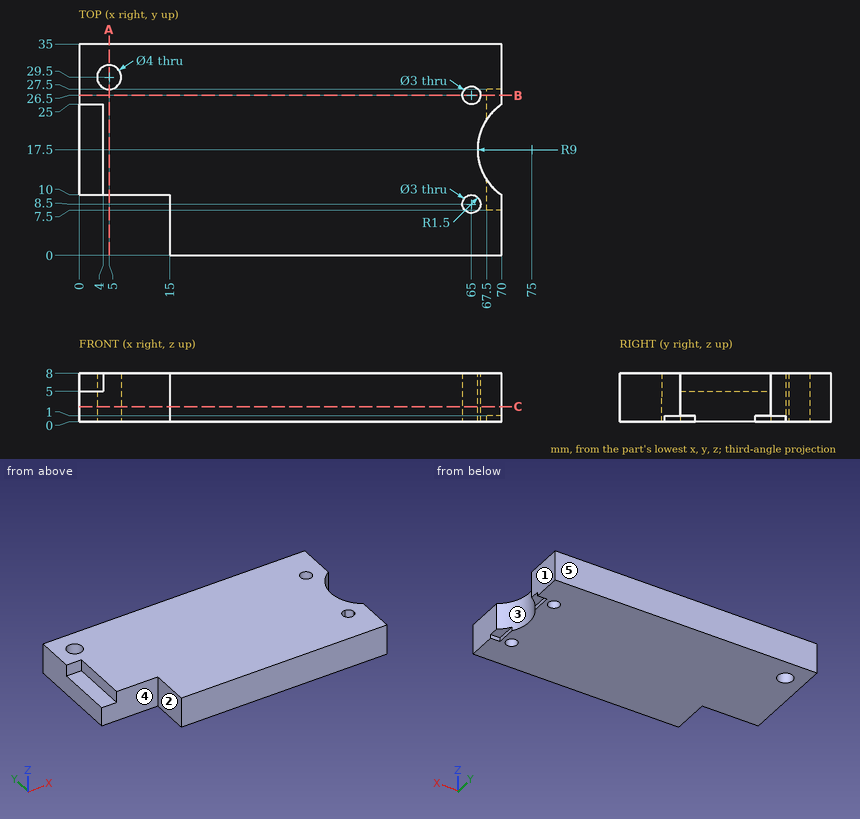
Study the drawing (mm; zero at the part's minimum x, y, z) and answer. A direction names the side the tool comes from. Give positions to 0.01 mm unless a question says otherwise; leave off trailing zeros. Order: outer loops, then holes, each group sorted by start corner. A loop starts at its lowest first (then second) coordinate and runs counter-clockwise, first axis right, second up. Notation, with made-up numbers: (51, 77.5) - (91, 77.5) arc R30 ccw to (91, 103.5) - close; hole circle Ø8 at (24, 76.5). An arc over 180 degrees is marked (long way). Use one line per item in the form item = value. Start each with the question number.
(1) For the marked faces 1 and 2, determine the directions among +Z, -Z, +X, -X, +Y, -Y from which every point of the face is accessible in a straight line to the end or side of a thin tool.
(2) A cutting plane is placed at C-C, the plane z = 2.5. Write down the section's boundary in (x, y), then the cut area to 3 significant figures.
(3) A cutting plane is placed at B-B, the plane y = 26.5. Write down the section's boundary in (x, z), then the cut area to 4 significant figures.
(4) A cutting plane is placed at A-A, the plane x = 5. Write down the section's boundary in (y, z), then the cut area to 3 significant figures.
(5) Flat-ended cylindrical pins translate along their axes: pin 1 Ø2.5 at (x, z) = (3, 6) entering from -Y; pin 2 Ø1.2 at (x, y) = (68.5, 24.5) entering from -Z; pin 3 Ø0.8 at (y, z) = (25.5, 0.5) entering from +X. Find the tip coordinate at first contact, or state that the pin passes through.
(6) Consider line 1 (Y direction, x = 65, z = 3); line 2 (X direction, y = 26.5, z = 5.75); line 3 (X direction, y = 8.5, z = 1.3). Determine where each line is inside the solid, lowest interval first. Write a range as from..to.
(7) The mould has two halves that part along Y. Classify the marked faces 3, 4 and 5: released by +Y, released by -Y, zero draft, split by the parting line, or undercut.
Ans:
q1.face_1 = +Z, -Z, +X, +Y, -Y
q1.face_2 = +Z, -Z, -X, -Y
q2.outline = (0, 10) - (15, 10) - (15, 0) - (70, 0) - (70, 10.02) arc R9 cw to (70, 24.98) - (70, 35) - (0, 35) - close; hole circle Ø4 at (5, 29.5); hole circle Ø3 at (65, 8.5); hole circle Ø3 at (65, 26.5)
q2.area = 2,230 mm^2
q3.outline = (0, 0) - (63.5, 0) - (63.5, 8) - (0, 8) - close; (66.5, 0) - (67.5, 0) - (67.5, 1) - (70, 1) - (70, 8) - (66.5, 8) - close
q3.area = 533.5 mm^2
q4.outline = (10, 0) - (27.5, 0) - (27.5, 8) - (10, 8) - close; (31.5, 0) - (35, 0) - (35, 8) - (31.5, 8) - close
q4.area = 168 mm^2
q5.pin_1 = 10
q5.pin_2 = 1
q5.pin_3 = 67.5
q6.line_1 = 0..7, 10..25, 28..35
q6.line_2 = 0..63.5, 66.5..70
q6.line_3 = 15..63.5, 66.5..70
q7.face_3 = undercut
q7.face_4 = released by -Y
q7.face_5 = released by +Y
